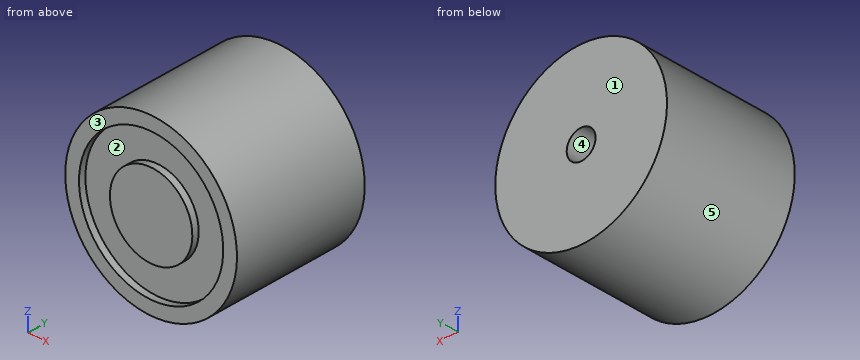
```python
from build123d import *

# Parameters (mm, degrees)
SKETCH_1_R          = 12.5
EXTRUDE_1_DEPTH     = 20
SKETCH_2_R          = 10.5
SKETCH_2_R_2        = 6
CUT_EXTRUDE_1_DEPTH = 1
SKETCH_3_R          = 2.1
CUT_EXTRUDE_2_DEPTH = 10


with BuildPart() as part:
    # 草图1 → 凸台-拉伸1 (new body)
    with BuildSketch(Plane(origin=(0, 0, 0), x_dir=(1, 0, 0), z_dir=(0, 1, 0))):
        with Locations(Location((0, 0, 0), (0, 0, 270))):
            Circle(SKETCH_1_R)
    extrude(amount=EXTRUDE_1_DEPTH)

    # 草图2 → 切除-拉伸1 (cut)
    with BuildSketch(Plane.XZ):
        with Locations(Location((0, 0, 0), (0, 0, 270))):
            Circle(SKETCH_2_R)
        with Locations(Location((0, 0, 0), (0, 0, 270))):
            Circle(SKETCH_2_R_2, mode=Mode.SUBTRACT)
    extrude(amount=-CUT_EXTRUDE_1_DEPTH, mode=Mode.SUBTRACT)

    # 草图3 → 切除-拉伸2 (cut)
    with BuildSketch(Plane(origin=(0, 20, 0), x_dir=(1, 0, 0), z_dir=(0, 1, 0))):
        with Locations(Location((0, 0, 0), (0, 0, 270))):
            Circle(SKETCH_3_R)
    extrude(amount=-CUT_EXTRUDE_2_DEPTH, mode=Mode.SUBTRACT)


solid = part.part
```
Build history of the part. All positions in model axes, mm. Face numbers are marked on the shaded views. A direction names the side the tool comes from. Coordinates: 2 decimals unless noted, no trailing zeros. Write each loop counter-clockwise with the first axis right and the second up, starting at its lowest first coordinate (ties: lowest second). Pieces come first, ordered by that corner, then holes.
1. Drop flat-ended pins along their axis: pin 1 (4 mm diameter, centred on y = 10.5, z = 3, fed in from +X); pin 2 (1 mm diameter, centred on y = 6, z = 8, fed in from -X); pin 3 (1 mm diameter, centred on y = 16.5, z = 5.5, fed in from -X). Give the stop position or say it passes through.
Answer block:
pin 1: stops at x = 12.46
pin 2: stops at x = -10
pin 3: stops at x = -11.46
2. Band-saw the part on A-A, the plane x = 0. Give the cut face in (y, z).
Answer block:
outline: (0, -12.5) - (20, -12.5) - (20, -2.1) - (10, -2.1) - (10, 2.1) - (20, 2.1) - (20, 12.5) - (0, 12.5) - (0, 10.5) - (1, 10.5) - (1, 6) - (0, 6) - (0, -6) - (1, -6) - (1, -10.5) - (0, -10.5) - close
3. Band-saw the part on D-D, the plane x = 4. Give the cut face in (y, z).
Answer block:
outline: (0, -11.84) - (20, -11.84) - (20, 11.84) - (0, 11.84) - (0, 9.71) - (1, 9.71) - (1, 4.47) - (0, 4.47) - (0, -4.47) - (1, -4.47) - (1, -9.71) - (0, -9.71) - close
4. Drill centre lines: probe 1 along X at (y, z) = (0.7, 0); probe 2 along X at (y, z) = (15.5, 0); probe 3 along Y at (x, z) = (-2.25, 6). Where is each one in solid material? Low to high.
Answer block:
probe 1: x = -12.5 to -10.5, -6 to 6, 10.5 to 12.5
probe 2: x = -12.5 to -2.1, 2.1 to 12.5
probe 3: y = 1 to 20
5. 3-axis set-ups, long thin cutter, end or side, ignore diameter. For the marked faces 1 and 2: which of +Z, -Z, +X, -X, +Y, -Y reach the whole face in a straight line?
Answer block:
face 1: +Z, -Z, +X, -X, +Y
face 2: -Y
6. Band-saw the part on B-B, the plane z = 0. Give the cut face in (x, y), and give its area (3 significant figures).
Answer block:
outline: (-12.5, 0) - (-10.5, 0) - (-10.5, 1) - (-6, 1) - (-6, 0) - (6, 0) - (6, 1) - (10.5, 1) - (10.5, 0) - (12.5, 0) - (12.5, 20) - (2.1, 20) - (2.1, 10) - (-2.1, 10) - (-2.1, 20) - (-12.5, 20) - close
area: 449 mm2
7. Pull direction Z, two halves, no side cores. Call the marked faces 3, 4 and 5: released by +Z, released by -Z, zero draft, split by the parting line, or undercut.
Answer block:
face 3: zero draft
face 4: undercut
face 5: split by the parting line
8. Band-saw the part on C-C, the plane y = 16.25. Give the cut face in (x, z).
Answer block:
outline: circle Ø25 at (0, 0); hole circle Ø4.2 at (0, 0)
